Source: CAD feature listing. Evaluate the final solid. Frame: model axes, mm. A direction names the side the tool comes from. Give positions to 0.01 mm unless a question says otherwise; leave off trailing zeros. Order: outer loops, then holes, each group sorted by start corner. A loop starts at its lowest first (then second) coordinate and runs counter-clockwise, first axis right, second up. Notation, with made-up numbers: M 41,9.25 L 72,9.25 A19 cw 72,46.25 Z; hole C 55.5,66.25 d4. An arc over 180 degrees is marked long. Use CSV: the item, a comma, the result in double quotes. Start each with the question number.
Item 1: First-contact query: pin 1 (4 mm diameter, centred on x = 5, z = -1.5, fed in from -Y); pin 2 (2 mm diameter, centred on y = 11, z = 4, fed in from -X); pin 3 (11 mm diameter, centred on x = -6.5, y = 18.5, fed in from +Z); pin 4 (2.5 mm diameter, centred on x = -1.5, z = 1.5, fed in from -Y). Flat tips, straight axial feed; report the tip coordinate or a pass-through.
Item 2: Section query C-C on y = 7.25. Return loops of the section in (x, z), and give its area (3 significant figures).
Item 3: Section query D-D on x = -2. Return loops of the section in (y, z).
Item 4: Pull-direction query (Z, two-part tool) for faces 1 (the face through (0, 0, 5)), 2 (the face through (10.161, 12.325, 4.213)), 3 (the face through (0, 14, -7.75)); classes: +Z half, -Z half, draft (parallel to the pull), parting line (faces both ways), or undercut.
Item 5: Section query B-B on z = -2. Return loops of the section in (x, y), and give its area (3 significant figures).
Item 6: Ray query, probe 1 along Z at (x, y) = (0, 2.3); probe 2 along Y at (x, z) = (1.5, -5.25); probe 3 along Y at (x, z) = (-7.25, -5.5). Return the intervals inside material, ascending. Write a range as from..to.
Item 7: Access query for faces 4 (the face through (5, 25, 0)), 5 (the face through (-7, 14.5, -6)), 6 (the face through (0, 19, -6)), 7 (the face through (0, 5, 0)), 8 (the face through (-6, 21, 4.25)). Directions: +Z, -Z, +X, -X, +Y, -Y. A direction counts if a zero-diameter tool reaches every point of the face in a straight line with its end or side. Return the directions, or none.
Item 8: Section query A-A on x = 2.25. Return loops of the section in (y, z).
from build123d import *

# Parameters (mm, degrees)
CROQUIS1_R              = 11
SALIENTE_EXTRUIR1_DEPTH = 25
CROQUIS2_R              = 4.25
CORTAR_EXTRUIR1_DEPTH   = 5
CROQUIS3_R              = 4.25
CORTAR_EXTRUIR2_DEPTH   = 6
CROQUIS5_W              = 8.5
CROQUIS5_H              = 15.5
CORTAR_EXTRUIR8_DEPTH   = 10
CORTAR_EXTRUIR16_DEPTH  = 12


with BuildPart() as part:
    # Croquis1 → Saliente-Extruir1 (new body)
    with BuildSketch(Plane(origin=(0, 0, 0), x_dir=(1, 0, 0), z_dir=(0, 1, 0))):
        Circle(CROQUIS1_R)
    extrude(amount=SALIENTE_EXTRUIR1_DEPTH)

    # Croquis2 → Cortar-Extruir1 (cut)
    with BuildSketch(Plane.XZ):
        Circle(CROQUIS2_R)
    extrude(amount=-CORTAR_EXTRUIR1_DEPTH, mode=Mode.SUBTRACT)

    # Croquis3 → Cortar-Extruir2 (cut)
    with BuildSketch(Plane(origin=(0, 25, 0), x_dir=(1, 0, 0), z_dir=(0, 1, 0))):
        Circle(CROQUIS3_R)
    extrude(amount=-CORTAR_EXTRUIR2_DEPTH, mode=Mode.SUBTRACT)

    # Croquis5 → Cortar-Extruir8 (cut)
    with BuildSketch(Plane(origin=(0, 19, 0), x_dir=(1, 0, 0), z_dir=(0, 1, 0))):
        Rectangle(CROQUIS5_W, CROQUIS5_H)
    extrude(amount=-CORTAR_EXTRUIR8_DEPTH, mode=Mode.SUBTRACT)

    # Croquis9 → Cortar-Extruir16 (cut, through all)
    with BuildSketch(Plane(origin=(0, 0, 0), x_dir=(0, 0, -1), z_dir=(1, 0, 0))):
        Polygon((-7.75, 9), (7.75, 9), (7.75, 14.5), (4.25, 14.5), (4.25, 25.5), (-4.25, 25.5), (-4.25, 14.5), (-7.75, 14.5), align=None)
    extrude(amount=-CORTAR_EXTRUIR16_DEPTH, mode=Mode.SUBTRACT)


solid = part.part
Verdict:
1,pin 1,"y = 0"
1,pin 2,"x = 4.25"
1,pin 3,"z = 10.95"
1,pin 4,"y = 5"
2,outline,"C 0,0 d22"
2,area,"380 mm2"
3,outline,"M 0,-10.82 L 25,-10.82 L 25,-4.25 L 19,-4.25 L 19,-7.75 L 9,-7.75 L 9,7.75 L 19,7.75 L 19,4.25 L 25,4.25 L 25,10.82 L 0,10.82 L 0,3.75 L 5,3.75 L 5,-3.75 L 0,-3.75 Z"
4,face 1,"draft"
4,face 2,"parting line"
4,face 3,"undercut"
5,outline,"M -10.82,0 L -3.75,0 L -3.75,5 L 3.75,5 L 3.75,0 L 10.82,0 L 10.82,25 L 3.75,25 L 3.75,19 L 4.25,19 L 4.25,9 L -10.82,9 Z"
5,area,"265 mm2"
6,probe 1,"-11..-4.25, 4.25..11"
6,probe 2,"0..9, 19..25"
6,probe 3,"0..9, 14.5..25"
7,face 4,"+Z, -Z, +X, -X, +Y"
7,face 5,"-X"
7,face 6,"none"
7,face 7,"-Y"
7,face 8,"-X, +Y"
8,outline,"M 0,-10.77 L 25,-10.77 L 25,-3.61 L 19,-3.61 L 19,-7.75 L 9,-7.75 L 9,7.75 L 19,7.75 L 19,3.61 L 25,3.61 L 25,10.77 L 0,10.77 L 0,3.61 L 5,3.61 L 5,-3.61 L 0,-3.61 Z"
